from build123d import *

# Parameters (mm, degrees)
SKETCH1_W                                  = 50.8
SKETCH1_H                                  = 22.352
BOSS_EXTRUDE1_DEPTH                        = 50.8
CUT_EXTRUDE2_DEPTH                         = 76.238898876
CUT_EXTRUDE2_DEPTH_BACK                    = 76.238898876
F_17_64_0_26563_DIAMETER_HOLE1_D           = 6.747002
F_17_64_0_26563_DIAMETER_HOLE1_ON_FACE_2_D = 6.747002


with BuildPart() as part:
    # Sketch1 → Boss-Extrude1 (new body)
    with BuildSketch(Plane(origin=(0, 0, 0), x_dir=(1, 0, 0), z_dir=(0, 1, 0))):
        with Locations((25.4, 11.176)):
            Rectangle(SKETCH1_W, SKETCH1_H)
    extrude(amount=BOSS_EXTRUDE1_DEPTH)

    # Sketch2 → Cut-Extrude2 (cut, two sides: drawn at the far end of the back side and taken through both)
    with BuildSketch(Plane.XY.offset(-CUT_EXTRUDE2_DEPTH_BACK)):
        Polygon((4.572, 198.1705643), (4.572, 50.8), (4.572, 4.572), (50.8, 4.572), (198.1705643, 4.572), (406.584015027, 212.985450727), (212.985450727, 406.584015027), align=None)
    extrude(amount=CUT_EXTRUDE2_DEPTH + CUT_EXTRUDE2_DEPTH_BACK, mode=Mode.SUBTRACT)

    # 17/64 (0.26563) Diameter Hole1 (through all)
    with Locations(Plane(origin=(4.572, 12.374496691, -11.175999046), x_dir=(0, 0, 1), z_dir=(1, 0, 0))):
        with Locations((0, 0), (-9.54e-07, -25.904093129)):
            Hole(F_17_64_0_26563_DIAMETER_HOLE1_D / 2)

    # 17/64 (0.26563) Diameter Hole1 on face 2 (through all)
    with Locations(Plane(origin=(12.343199837, 4.572, -11.175998262), x_dir=(0, 0, 1), z_dir=(0, 1, 0))):
        with Locations((0, 0), (-1.738e-06, 25.906798937)):
            Hole(F_17_64_0_26563_DIAMETER_HOLE1_ON_FACE_2_D / 2)


solid = part.part
Design review of the part built by this model. Coordinates are the model's own, in mm. A direction names the side the tool comes from. Give positions to 0.01 mm unless a question says otherwise; leave off trailing zeros. Loops run counter-clockwise (first coordinate to the right, second up) from the corner with the lowest first, then second, coordinate; pieces in that order, holes last. Notation, with made-up numbers: M 58.5,53.5 L 69.5,53.5 A29 ccw 69.5,86.5 Z; hole C 49.25,78 d5. An arc over 180 degrees is marked long. Answer as a JSON object with one key per item and string values.
Item 1: Machinability: for faces 4 (the face through (3, 14, -22.352)), 5 (the face through (27, 4.572, -11)), which of the approach directions +Z, -Z, +X, -X, +Y, -Y give a long, thin tool a straight path to every point of the face, cutting with its end or side? Answer none if there is none.
Output values:
{"face 4": "-Z, +X, -X, +Y, -Y", "face 5": "+Z, -Z, +X, +Y"}
Item 2: For P1, Ø8, axis at y = 12.37, z = -11.18, coming from the +X side, flat-tipped, find the tip position at first contact; note if it passes through.
Output values:
{"P1": "stops at x = 4.57"}
Item 3: We need section D-D (y = 7.5). State the section outline as (x, z) points.
Output values:
{"outline": "M 0,-22.35 L 4.57,-22.35 L 4.57,0 L 0,0 Z"}
Item 4: We need section C-C (z = -2.5). State the section outline as (x, y) points.
Output values:
{"outline": "M 0,0 L 50.8,0 L 50.8,4.57 L 4.57,4.57 L 4.57,50.8 L 0,50.8 Z"}
Item 5: Mouldability with a two-part tool opening along Z and no side actions: class faces 1 (the face through (3, 14, 0)), 2 (the face through (2.254, 41.271, -12.733)), 3 (the face through (2, 50.8, -11)) as pulls with the +Z half, pulls with the -Z half, needs draft (parallel to the pull), parting line crosses it, or undercut.
Output values:
{"face 1": "pulls with the +Z half", "face 2": "undercut", "face 3": "needs draft"}
Item 6: Wall thickness on line 1 along X through (y, z) = (32, -10.5): over which ranges is the line inside the solid? List them lowest first.
Output values:
{"line 1": "x = 0 to 4.57"}
Item 7: We need section B-B (z = -13.75). State the section outline as (x, y) points.
Output values:
{"outline": "M 0,0 L 10.16,0 L 10.16,4.57 L 4.57,4.57 L 4.57,10.19 L 0,10.19 Z; M 0,14.56 L 4.57,14.56 L 4.57,36.1 L 0,36.1 Z; M 0,40.46 L 4.57,40.46 L 4.57,50.8 L 0,50.8 Z; M 14.52,0 L 36.07,0 L 36.07,4.57 L 14.52,4.57 Z; M 40.43,0 L 50.8,0 L 50.8,4.57 L 40.43,4.57 Z"}
Item 8: We need section A-A (x = 11). State the section outline as (y, z) points, and give its area (3 significant figures).
Output values:
{"outline": "M 0,-22.35 L 4.57,-22.35 L 4.57,-14.27 L 0,-14.27 Z; M 0,-8.08 L 4.57,-8.08 L 4.57,0 L 0,0 Z", "area": "73.9 mm2"}
